```python
from build123d import *

# Parameters (mm, degrees)
SKETCH1_W              = 900
SKETCH1_H              = 200
SKETCH1_R              = 5
BOSS_EXTRUDE1_DEPTH    = 15
SKETCH2_W              = 208
SKETCH2_H              = 126
SHREDDER_OPENING_DEPTH = 462.221205063
SKETCH3_W              = 170
SKETCH3_H              = 81.5
SKETCH3_R              = 5
LEGS_ADD_ON_DEPTH      = 15


with BuildPart() as part:
    # Sketch1 → Boss-Extrude1 (new body)
    with BuildSketch(Plane(origin=(0, 0, 0), x_dir=(1, 0, 0), z_dir=(0, 1, 0))):
        Rectangle(SKETCH1_W, SKETCH1_H)
        with Locations(Location((425, -75, 0), (0, 0, 270))):
            Circle(SKETCH1_R, mode=Mode.SUBTRACT)
        with Locations(Location((425, 75, 0), (0, 0, 270))):
            Circle(SKETCH1_R, mode=Mode.SUBTRACT)
        with Locations(Location((-425, -75, 0), (0, 0, 270))):
            Circle(SKETCH1_R, mode=Mode.SUBTRACT)
        with Locations(Location((-425, 75, 0), (0, 0, 270))):
            Circle(SKETCH1_R, mode=Mode.SUBTRACT)
    extrude(amount=-BOSS_EXTRUDE1_DEPTH)

    # Sketch2 → Shredder Opening (cut, through all)
    with BuildSketch(Plane.XZ.offset(15)):
        with Locations((-275, 7.5)):
            Rectangle(SKETCH2_W, SKETCH2_H)
    extrude(amount=-SHREDDER_OPENING_DEPTH, mode=Mode.SUBTRACT)

    # Sketch3 → Legs add on (add, through all)
    with BuildSketch(Plane(origin=(0, 0, 0), x_dir=(1, 0, 0), z_dir=(0, 1, 0))):
        with Locations((115, 140.75)):
            Rectangle(SKETCH3_W, SKETCH3_H)
        with Locations(Location((175, 156.5, 0), (0, 0, 270))):
            Circle(SKETCH3_R, mode=Mode.SUBTRACT)
        with Locations(Location((55, 156.5, 0), (0, 0, 90))):
            Circle(SKETCH3_R, mode=Mode.SUBTRACT)
    extrude(amount=-LEGS_ADD_ON_DEPTH)


solid = part.part
```
Geometry check sheet. Reference: the model listing, model coordinates, mm. A direction names the side the tool comes from. Coordinates: 2 decimals unless noted, no trailing zeros. Write each loop counter-clockwise with the first axis right and the second up, starting at its lowest first coordinate (ties: lowest second). Pieces come first, ordered by that corner, then holes. Notation, with made-up numbers: M -27,16.5 L -1,16.5 A34 ccw -1,51.5 Z; hole C 62.5,85.25 d5. An arc over 180 degrees is marked long. Answer as a JSON object with one key per item and string values.
1. Section check C-C, the plane y = -11. Enter the section's corners in (x, z), plus the area to 3 significant figures.
Answers below:
{"outline": "M -450,-100 L 30,-100 L 30,-181.5 L 200,-181.5 L 200,-100 L 450,-100 L 450,100 L -450,100 Z; hole C -425,-75 d10; hole C -425,75 d10; hole M -379,-55.5 L -171,-55.5 L -171,70.5 L -379,70.5 Z; hole C 55,-156.5 d10; hole C 175,-156.5 d10; hole C 425,-75 d10; hole C 425,75 d10", "area": "167,000 mm²"}
2. Section check A-A, the plane x = -274.5. Enter the section's corners in (y, z).
Answers below:
{"outline": "M -15,-100 L 0,-100 L 0,-55.5 L -15,-55.5 Z; M -15,70.5 L 0,70.5 L 0,100 L -15,100 Z"}
3. Scan lines: L1, parallel to X at y = -8.25, z = -75; L2, parallel to Z at x = 425, y = -9.5; L3, parallel to X at y = -3.5, z = -156.5. Record each from-to range of solid material in increasing order.
Answers below:
{"L1": "x = -450 to -430, -420 to 420, 430 to 450", "L2": "z = -100 to -80, -70 to 70, 80 to 100", "L3": "x = 30 to 50, 60 to 170, 180 to 200"}
4. Draft check along X on faces 4 (the flat face through (30, -7, -140)), 5 (the flat face through (-213, -7, -100)), 6 (the flat face through (-379, -8, 7)), 7 (the flat face through (450, -7, 1)). Enter one of: released by +X, released by -X, zero draft, split by the parting line, or undercut.
Answers below:
{"face 4": "released by -X", "face 5": "zero draft", "face 6": "undercut", "face 7": "released by +X"}
5. Go/stop test with flat-tipped pins: pin 1 Ø2 at (x, y) = (340.5, -11.5) entering from -Z; pin 2 Ø4.5 at (y, z) = (-9, -129.5) entering from +X; pin 3 Ø4.5 at (y, z) = (-5, -137.5) entering from -X. Record where each tip stops, or that it passes through.
Answers below:
{"pin 1": "stops at z = -100", "pin 2": "stops at x = 200", "pin 3": "stops at x = 30"}
6. Section check B-B, the plane z = -43.5. Enter the section's corners in (x, y).
Answers below:
{"outline": "M -450,-15 L -379,-15 L -379,0 L -450,0 Z; M -171,-15 L 450,-15 L 450,0 L -171,0 Z"}
7. Section check D-D, the plane x = 236.5. Enter the section's corners in (y, z), plus the area to 3 significant figures.
Answers below:
{"outline": "M -15,-100 L 0,-100 L 0,100 L -15,100 Z", "area": "3,000 mm²"}
8. Tool access check on faces 1 (the flat face through (-276, -8, 70.5)), 2 (the flat face through (-450, -7, 1)), 3 (the flat face through (323, -7, -100)). Record the directions out of +Z, -Z, +X, -X, +Y, -Y that give a thin tool (end or side, any length) a straight path to the whole face; none if there is none.
Answers below:
{"face 1": "+Y, -Y", "face 2": "+Z, -Z, -X, +Y, -Y", "face 3": "-Z, +X, +Y, -Y"}
